Here's how the part is built. I have some questions about the finished solid (model axes, mm). Face numbers are marked on the shaded views. A direction names the side the tool comes from. Round coordinates to 2 decimals unless told otherwise and drop trailing zeros. Order: outer loops, then holes, each group sorted by start corner. A loop starts at its lowest first (then second) coordinate and runs counter-clockwise, first axis right, second up. Notation, with made-up numbers: M -34.75,31.5 L -6.75,31.5 A24 cw -6.75,68.5 Z; hole C 26.5,-32 d4. An arc over 180 degrees is marked long. Write item = value, one per line. Start each with the question number.
Item 1: For the marked faces 1, 2 and 3, which set-ups out of +Z, -Z, +X, -X, +Y, -Y let a thin tool reach every point of the face, with its end or its side?
Item 2: Please list where these lines run through material, in increasing order: L1, parallel to Y at x = 68.5, z = -21.5; L2, parallel to X at y = 24, z = 8; L3, parallel to X at y = 11.75, z = 8.
Item 3: I'm going to push flat-ended pins straight in: P1, Ø12.5, axis at y = 12.5, z = -16.5, coming from the -X side; P2, Ø4, axis at y = 16.5, z = -10.5, coming from the +X side; P3, Ø1.7, axis at y = 19, z = 0, coming from the +X side. Where does each tip first touch, or does it pass through?
Item 4: I want a section at A-A, the plane y = 19.5. List the corners of the cut face in (x, z) for me.
Item 5: I want a section at C-C, the plane x = -70.5. List the corners of the cut face in (y, z) for me, plus the area to 3 significant figures.
```python
from build123d import *

# Parameters (mm, degrees)
SKETCH1_W           = 63.5
SKETCH1_H           = 63.5
BOSS_EXTRUDE1_DEPTH = 25.4
SKETCH1_3_W         = 63.5
SKETCH1_3_H         = 63.5
BOSS_EXTRUDE2_DEPTH = 2.54
SKETCH1_4_W         = 127
SKETCH1_4_H         = 63.5
BOSS_EXTRUDE3_DEPTH = 2.54
CHAMFER2_SIZE       = 25.4
FILLET1_R           = 25.4


with BuildPart() as part:
    # Sketch1 → Boss-Extrude1 (new body)
    with BuildSketch(Plane(origin=(0, 0, 0), x_dir=(1, 0, 0), z_dir=(0, 1, 0))):
        Rectangle(SKETCH1_W, SKETCH1_H)
        Polygon((-0.79375, 25.4), (-0.79375, 0.79375), (-25.4, 0.79375), (-25.4, -0.79375), (-0.79375, -0.79375), (-0.79375, -25.4), (0.79375, -25.4), (0.79375, -0.79375), (25.4, -0.79375), (25.4, 0.79375), (0.79375, 0.79375), (0.79375, 25.4), align=None, mode=Mode.SUBTRACT)
    extrude(amount=BOSS_EXTRUDE1_DEPTH)

    # Sketch1<3> → Boss-Extrude2 (add)
    with BuildSketch(Plane(origin=(0, 0, 0), x_dir=(1, 0, 0), z_dir=(0, 1, 0))):
        Rectangle(SKETCH1_3_W, SKETCH1_3_H)
    extrude(amount=-BOSS_EXTRUDE2_DEPTH)

    # Sketch1<4> → Boss-Extrude3 (add)
    with BuildSketch(Plane(origin=(0, 0, 0), x_dir=(1, 0, 0), z_dir=(0, 1, 0))):
        with Locations((95.25, 0)):
            Rectangle(SKETCH1_4_W, SKETCH1_4_H)
        with Locations((-95.25, 0)):
            Rectangle(SKETCH1_4_W, SKETCH1_4_H)
    extrude(amount=-BOSS_EXTRUDE3_DEPTH)

    # Chamfer2
    chamfer2_edges = [part.edges().sort_by_distance(p)[0] for p in [
        (31.75, 0, 0),
        (-31.75, 0, 0),
    ]]
    chamfer(chamfer2_edges, length=CHAMFER2_SIZE - 0.0001)  # a hair under: the kernel refuses the full size

    # Fillet1
    fillet1_edges = [part.edges().sort_by_distance(p)[0] for p in [
        (158.75, -1.27, -31.75),
        (158.75, -1.27, 31.75),
        (-158.75, -1.27, -31.75),
        (-158.75, -1.27, 31.75),
    ]]
    fillet(fillet1_edges, radius=FILLET1_R)


solid = part.part
```
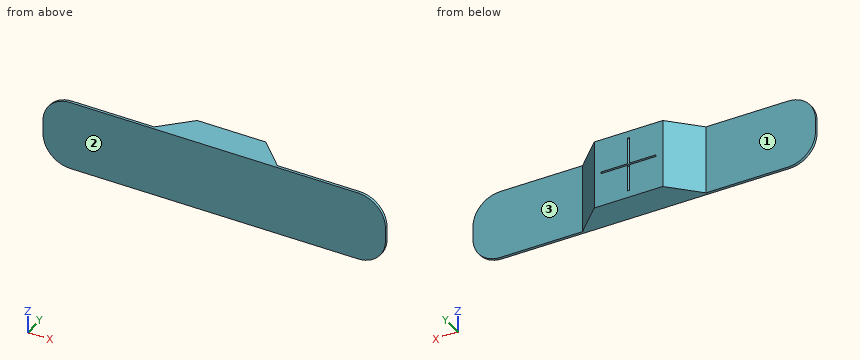
Filled in:
q1.face_1 = +Z, -Z, -X, +Y
q1.face_2 = +Z, -Z, +X, -X, -Y
q1.face_3 = +Z, -Z, +X, +Y
q2.L1 = -2.54 to 0
q2.L2 = -33.15 to -0.79, 0.79 to 33.15
q2.L3 = -45.4 to -0.79, 0.79 to 45.4
q3.P1 = -50.9
q3.P2 = 42.65
q3.P3 = 39
q4.outline = M -37.65,-31.75 L 37.65,-31.75 L 37.65,31.75 L -37.65,31.75 Z; hole M -25.4,-0.79 L -0.79,-0.79 L -0.79,-25.4 L 0.79,-25.4 L 0.79,-0.79 L 25.4,-0.79 L 25.4,0.79 L 0.79,0.79 L 0.79,25.4 L -0.79,25.4 L -0.79,0.79 L -25.4,0.79 Z
q5.outline = M -2.54,-31.75 L 0,-31.75 L 0,31.75 L -2.54,31.75 Z
q5.area = 161 mm^2
